The figure shows three views and two pictorial views of one solid part (mm, origin at its lowest corner). Answer the questions. Coordinates: 2 decimals unless noted, no trailing zeros. Order: outer loops, then holes, each group sorted by start corner. A loop starts at its lowest first (then second) coordinate and runs counter-clockwise, first axis right, second up. Notation, with made-up numbers: (73, -29) -> (122, -29) arc R24 ccw to (122, -1) -> close; hole circle Ø8 at (40, 86.25). An arc over 180 degrees is marked (long way). Return JSON: item names as keys, results as strings. Group by question number.
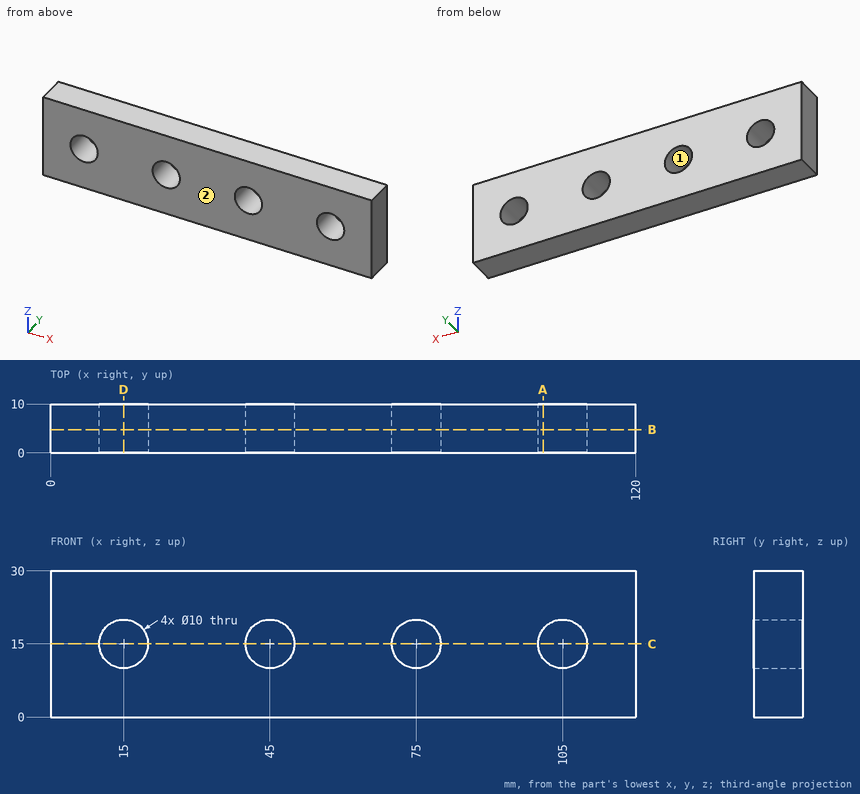
1. Find section C-C on z = 15. Determine the outline of the cut face in (x, y), and give its area (3 significant figures).
2. Straight lines are drawn through the part: L1, parallel to X at y = 5.25, z = 15; L2, parallel to X at y = 9.25, z = 16.25; L3, parallel to Z at x = 105, y = 4.5. For each, find the intervals that lie inside material, in ascending order.
3. For a pull along X with two mould halves and no side action, classify the marked faces 1 and 2 as released by +X, released by -X, zero draft, split by the parting line, or undercut.
4. Given pin 1 (8 mm diameter, centred on x = 75, z = 15, fed in from +Y), flat-ended and moving along its own axis, determine where the tip first touches the part or whether it passes through.
5. Find section B-B on y = 4.75. Determine the outline of the cut face in (x, z).
6. Find section A-A on x = 101. Determine the outline of the cut face in (y, z).
7. Find section D-D on x = 15. Determine the outline of the cut face in (y, z), and give its area (3 significant figures).
Result:
{
 "1": {"outline": "(0, 0) -> (10, 0) -> (10, 10) -> (0, 10) -> close; (20, 0) -> (40, 0) -> (40, 10) -> (20, 10) -> close; (50, 0) -> (70, 0) -> (70, 10) -> (50, 10) -> close; (80, 0) -> (100, 0) -> (100, 10) -> (80, 10) -> close; (110, 0) -> (120, 0) -> (120, 10) -> (110, 10) -> close", "area": "800 mm^2"},
 "2": {"L1": "0 to 10, 20 to 40, 50 to 70, 80 to 100, 110 to 120", "L2": "0 to 10.16, 19.84 to 40.16, 49.84 to 70.16, 79.84 to 100.16, 109.84 to 120", "L3": "0 to 10, 20 to 30"},
 "3": {"face 1": "undercut", "face 2": "zero draft"},
 "4": {"pin 1": "through"},
 "5": {"outline": "(0, 0) -> (120, 0) -> (120, 30) -> (0, 30) -> close; hole circle Ø10 at (15, 15); hole circle Ø10 at (45, 15); hole circle Ø10 at (75, 15); hole circle Ø10 at (105, 15)"},
 "6": {"outline": "(0, 0) -> (10, 0) -> (10, 12) -> (0, 12) -> close; (0, 18) -> (10, 18) -> (10, 30) -> (0, 30) -> close"},
 "7": {"outline": "(0, 0) -> (10, 0) -> (10, 10) -> (0, 10) -> close; (0, 20) -> (10, 20) -> (10, 30) -> (0, 30) -> close", "area": "200 mm^2"}
}
